```python
from build123d import *

# Parameters (mm, degrees)
F0_R     = 5.08
F1_DEPTH = 6.35
F2_R     = 3.175
F3_DEPTH = 25.4


with BuildPart() as f1:
    # F0 (on Front) → F1 (new body)
    with BuildSketch(Plane.XZ):
        with BuildLine():
            Line((-32.902092, -5.197908), (-8.980256, -29.119744))
            ThreePointArc((-8.980256, -29.119744), (0, -32.839488), (8.980256, -29.119744))
            Line((8.980256, -29.119744), (32.902092, -5.197908))
            ThreePointArc((32.902092, -5.197908), (34.67947, -1.728008), (34.094357, 2.126459))
            ThreePointArc((34.094357, 2.126459), (0, 23.221024), (-34.094357, 2.126459))
            ThreePointArc((-34.094357, 2.126459), (-34.67947, -1.728008), (-32.902092, -5.197908))
        make_face()
        with Locations((0, -23.374978)):
            Circle(F0_R, mode=Mode.SUBTRACT)
    extrude(amount=F1_DEPTH)

    # F2 (on face) → F3 (cut)
    with BuildSketch(Plane.XZ.offset(6.35)):
        with Locations((-31.760779, 8.385801)):
            Circle(F2_R)
        with Locations((-24.65719, 15.813367)):
            Circle(F2_R)
        with Locations((-15.873253, 21.149301)):
            Circle(F2_R)
        with Locations((-6.007581, 24.029968)):
            Circle(F2_R)
        with Locations((4.267498, 24.259054)):
            Circle(F2_R)
        with Locations((14.251754, 21.820948)):
            Circle(F2_R)
        with Locations((23.264776, 16.881804)):
            Circle(F2_R)
        with Locations((30.692343, 9.778214)):
            Circle(F2_R)
    extrude(amount=-F3_DEPTH, mode=Mode.SUBTRACT)


solid = f1.part
```
Geometry check sheet. Reference: the model listing, model coordinates, mm. Coordinates: 2 decimals unless noted, no trailing zeros. Order: outer loops, then holes, each group sorted by start corner. A loop starts at its lowest first (then second) coordinate and runs counter-clockwise, first axis right, second up.
Item 1: Section check D-D (x = 12). Enter the section's corners in (y, z), plus the area to 3 significant figures.
Item 2: Depth check by flat-ended pin: pin 1 (1.5 mm diameter, centred on x = 10.5, y = -2, fed in from -Z). Enter the tip coordinate at first touch or a pass-through.
Item 3: Section check C-C (z = -8). Enter the section's corners in (x, y), plus the area to 3 significant figures.
Item 4: Mould release check, pull along X, two halves, no side actions. Record for faces 1 (the flat face through (20.8, -3.1, -17.3)), 2 (the cylindrical face through (-1.101, -3.131, -28.334)), 3 (the flat face through (-21.1, -3.1, -17)): released by +X, released by -X, zero draft, split by the parting line, or undercut.
Item 5: Section check A-A (x = 0). Enter the section's corners in (y, z), plus the area to 3 significant figures.
Item 6: Scan lines: line 1 along Z through (x, y) = (0, -3.5); line 2 along X through (y, z) = (-5, -26.5); line 3 along Z through (x, y) = (-1, -1.25). Record each from-to range of solid material in increasing order.
Check sheet entries:
1. outline: (-6.35, -26.1) - (0, -26.1) - (0, 19.58) - (-6.35, 19.58) - close
1. area: 290 mm2
2. pin 1: stops at z = -28.35
3. outline: (-30.1, -6.35) - (30.1, -6.35) - (30.1, 0) - (-30.1, 0) - close
3. area: 382 mm2
4. face 1: released by +X
4. face 2: undercut
4. face 3: released by -X
5. outline: (-6.35, -32.84) - (0, -32.84) - (0, -28.45) - (-6.35, -28.45) - close; (-6.35, -18.29) - (0, -18.29) - (0, 23.22) - (-6.35, 23.22) - close
5. area: 291 mm2
6. line 1: z = -32.84 to -28.45, -18.29 to 23.22
6. line 2: x = -11.6 to -4.01, 4.01 to 11.6
6. line 3: z = -32.8 to -28.36, -18.39 to 23.21
